The model under review builds one solid part; all positions refer to its coordinate system, in mm. Give positions to 0.01 mm unless a question says otherwise; leave off trailing zeros. Loops run counter-clockwise (first coordinate to the right, second up) from the corner with the lowest first, then second, coordinate; pieces in that order, holes last. Notation, with made-up numbers: M -11,44.5 L 31,44.5 A19 cw 31,74.5 Z; hole C -14.5,65.25 d7. An arc over 180 degrees is marked long. Write item = value, one per line. Start each with the question number.
1. Wall thickness on line 1 along X through (y, z) = (0.9, 5); line 2 along Z through (x, y) = (24, 1.2); line 3 along X through (y, z) = (1.65, -5): over which ranges is each line inside the solid? List them lowest first. Write a range as from..to.
2. We need section C-C on y = 2.55. Give the boundary of the cut face in (x, z), then the cut area to 3 significant figures.
3. We need section D-D on z = -5. Give the boundary of the cut face in (x, y), then the cut area to 3 significant figures.
4. We need section B-B on z = -0.5. Give the boundary of the cut face in (x, y), then the cut area to 3 significant figures.
5. For pin 1 (1.4 mm diameter, centred on x = 24, z = -5, fed in from +Y), flat-tipped, find the tip position at first contact; note if it passes through.
6. We need section A-A on x = 1. Give the boundary of the cut face in (y, z), then the cut area to 3 significant figures.
from build123d import *

# Parameters (mm, degrees)
SKETCH1_W           = 55
SKETCH1_H           = 34
SKETCH1_R           = 1.1
SKETCH1_R_2         = 1.3
SKETCH1_R_3         = 1.2
SKETCH1_R_4         = 1.4
SKETCH1_W_2         = 43
SKETCH1_H_2         = 22
BOSS_EXTRUDE1_DEPTH = 3


with BuildPart() as part:
    # Sketch1 → Boss-Extrude1 (new body)
    with BuildSketch(Plane(origin=(0, 0, 0), x_dir=(1, 0, 0), z_dir=(0, 1, 0))):
        Rectangle(SKETCH1_W, SKETCH1_H)
        with Locations((-24, 5)):
            Circle(SKETCH1_R, mode=Mode.SUBTRACT)
        with Locations((-24, -5)):
            Circle(SKETCH1_R_2, mode=Mode.SUBTRACT)
        with Locations((24, 5)):
            Circle(SKETCH1_R_3, mode=Mode.SUBTRACT)
        with Locations((24, -5)):
            Circle(SKETCH1_R_4, mode=Mode.SUBTRACT)
        Rectangle(SKETCH1_W_2, SKETCH1_H_2, mode=Mode.SUBTRACT)
    extrude(amount=BOSS_EXTRUDE1_DEPTH)


solid = part.part
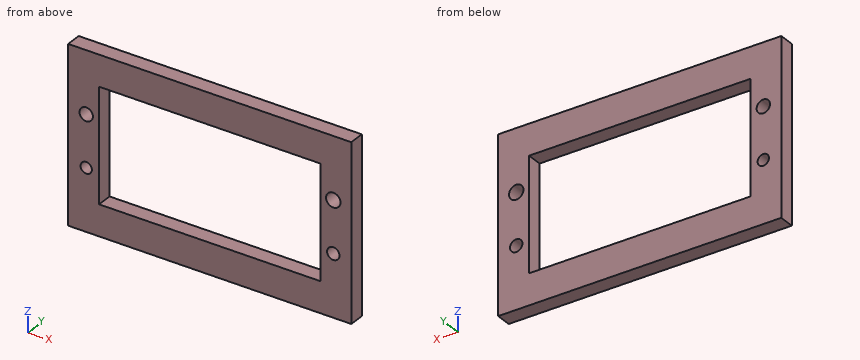
Final values:
q1.line_1 = -27.5..-25.3, -22.7..-21.5, 21.5..22.6, 25.4..27.5
q1.line_2 = -17..-6.2, -3.8..3.6, 6.4..17
q1.line_3 = -27.5..-25.1, -22.9..-21.5, 21.5..22.8, 25.2..27.5
q2.outline = M -27.5,-17 L 27.5,-17 L 27.5,17 L -27.5,17 Z; hole C -24,5 d2.6; hole C -24,-5 d2.2; hole M -21.5,-11 L 21.5,-11 L 21.5,11 L -21.5,11 Z; hole C 24,5 d2.8; hole C 24,-5 d2.4
q2.area = 904 mm²
q3.outline = M -27.5,0 L -25.1,0 L -25.1,3 L -27.5,3 Z; M -22.9,0 L -21.5,0 L -21.5,3 L -22.9,3 Z; M 21.5,0 L 22.8,0 L 22.8,3 L 21.5,3 Z; M 25.2,0 L 27.5,0 L 27.5,3 L 25.2,3 Z
q3.area = 22.2 mm²
q4.outline = M -27.5,0 L -21.5,0 L -21.5,3 L -27.5,3 Z; M 21.5,0 L 27.5,0 L 27.5,3 L 21.5,3 Z
q4.area = 36.0 mm²
q5.pin_1 = through
q6.outline = M 0,-17 L 3,-17 L 3,-11 L 0,-11 Z; M 0,11 L 3,11 L 3,17 L 0,17 Z
q6.area = 36.0 mm²
